from build123d import *

# Parameters (mm, degrees)
F1_DEPTH = 25.4


with BuildPart() as f1:
    # F0 (on Front) → F1 (new body)
    with BuildSketch(Plane.XZ):
        Polygon((-130.822942, -63.342907), (0, 0), (-53.333733, 35.463728), align=None)
        Polygon((-53.333733, 35.463728), (0, 0), (126.89946, 44.269524), (90.807401, 68.268575), align=None)
    extrude(amount=F1_DEPTH)


solid = f1.part
Verification items for the finished model (mm, model axes). Give positions to 0.01 mm unless a question says otherwise; leave off trailing zeros. Order: outer loops, then holes, each group sorted by start corner. A loop starts at its lowest first (then second) coordinate and runs counter-clockwise, first axis right, second up. Notation, with made-up numbers: M -21.75,-23 L -5.75,-23 A13 ccw -5.75,-7 Z; hole C 3.5,-34 d7. An arc over 180 degrees is marked long. Answer as a JSON object with one key per item and string values. Group by question number.
1) Scan lines: line 1 along Z through (x, y) = (-79, -17.25); line 2 along Z through (x, y) = (92, -14.75); line 3 along X through (y, z) = (-9, -10). Record each from-to range of solid material in increasing order. Write a range as [from, to].
2) Cross-section at B-B (x = 55.5). Enter the section's corners in (y, z).
3) Depth check by flat-ended pin: pin 1 Ø8 at (y, z) = (-11.5, -31) entering from -X (3 decimals); pin 2 Ø8 at (y, z) = (-4.5, 37) entering from -X; pin 3 Ø4 at (x, y) = (-13.5, -11) entering from -Z. Enter the tip coordinate at first touch or a pass-through.
4) Cross-section at A-A (y = -21.25). Enter the section's corners in (x, z).
5) Cross-section at C-C (z = 3.5). Enter the section's corners in (x, y), then the cut area to 3 significant figures.
Result sheet:
{
 "1": {"line 1": "z = [-38.25, 2.74]", "line 2": "z = [32.09, 67.48]", "line 3": "x = [-88.99, -20.65]"},
 "2": {"outline": "M -25.4,19.36 L 0,19.36 L 0,60.23 L -25.4,60.23 Z"},
 "3": {"pin 1": "stops at x = -108.595", "pin 2": "stops at x = -55.27", "pin 3": "stops at z = -7.5"},
 "4": {"outline": "M -130.82,-63.34 L 0,0 L 126.9,44.27 L 90.81,68.27 L -53.33,35.46 Z"},
 "5": {"outline": "M -78.4,-25.4 L 10.03,-25.4 L 10.03,0 L -78.4,0 Z", "area": "2,250 mm2"}
}
